```python
from build123d import *

# Parameters (mm, degrees)
SKETCH1_W           = 190
SKETCH1_H           = 114
BOSS_EXTRUDE1_DEPTH = 2.5
SKETCH3_R           = 2
CUT_EXTRUDE2_DEPTH  = 10
SKETCH4_W           = 23
SKETCH4_H           = 13
CUT_EXTRUDE3_DEPTH  = 21


with BuildPart() as part:
    # Sketch1 → Boss-Extrude1 (new body)
    with BuildSketch(Plane.XY):
        Rectangle(SKETCH1_W, SKETCH1_H)
    extrude(amount=BOSS_EXTRUDE1_DEPTH)

    # Sketch3 → Cut-Extrude2 (cut)
    with BuildSketch(Plane.XY.offset(2.5)):
        with Locations((-90, 52)):
            Circle(SKETCH3_R)
        with Locations((90, 52)):
            Circle(SKETCH3_R)
        with Locations((90, -52)):
            Circle(SKETCH3_R)
        with Locations((-90, -52)):
            Circle(SKETCH3_R)
    extrude(amount=-CUT_EXTRUDE2_DEPTH, mode=Mode.SUBTRACT)

    # Sketch4 → Cut-Extrude3 (cut)
    with BuildSketch(Plane.XY.offset(2.5)):
        with Locations((57.5, -39)):
            Rectangle(SKETCH4_W, SKETCH4_H)
    extrude(amount=-CUT_EXTRUDE3_DEPTH, mode=Mode.SUBTRACT)


solid = part.part
```
Work out the finished part from the listing and answer in its coordinate system (mm). Coordinates: 2 decimals unless noted, no trailing zeros. Write each loop counter-clockwise with the first axis right and the second up, starting at its lowest first coordinate (ties: lowest second). Pieces come first, ordered by that corner, then holes.
Q1. A cutting plane is placed at C-C, the plane z = 1.9. Give the vertices of the cut face in (x, y).
Q2. Find the intervals of material crossed by line 1 (Y direction, x = 90, z = 0.9); line 2 (Y direction, x = 56, z = 1.85), in increasing order.
Q3. A cutting plane is placed at D-D, the plane x = -90. Give the vertices of the cut face in (y, z).
Q4. Each of these flat-tipped pins is pushed along its axis until it touches: pin 1 Ø5 at (x, y) = (-90, -52) entering from -Z; pin 2 Ø3 at (x, y) = (90, 52) entering from -Z. Where does it stop, or does it pass through?
Q5. A cutting plane is placed at B-B, the plane y = -52. Give the vertices of the cut face in (x, z).
Q6. Determine the mould class of faces 1 (the face through (-1, 1, 0)), 2 (the face through (91.847, -52.766, 1.268)), 3 (the face through (91.847, 51.234, 1.268)) for opening direction X: released by +X, released by -X, zero draft, split by the parting line, or undercut.
Q7. A cutting plane is placed at A-A, the plane x = 60. Give the vertices of the cut face in (y, z), then the cut area to 4 significant figures.
Findings below:
1. outline: (-95, -57) - (95, -57) - (95, 57) - (-95, 57) - close; hole circle Ø4 at (-90, -52); hole circle Ø4 at (-90, 52); hole (46, -45.5) - (69, -45.5) - (69, -32.5) - (46, -32.5) - close; hole circle Ø4 at (90, -52); hole circle Ø4 at (90, 52)
2. line 1: y = -57 to -54, -50 to 50, 54 to 57
2. line 2: y = -57 to -45.5, -32.5 to 57
3. outline: (-57, 0) - (-54, 0) - (-54, 2.5) - (-57, 2.5) - close; (-50, 0) - (50, 0) - (50, 2.5) - (-50, 2.5) - close; (54, 0) - (57, 0) - (57, 2.5) - (54, 2.5) - close
4. pin 1: stops at z = 0
4. pin 2: passes through
5. outline: (-95, 0) - (-92, 0) - (-92, 2.5) - (-95, 2.5) - close; (-88, 0) - (88, 0) - (88, 2.5) - (-88, 2.5) - close; (92, 0) - (95, 0) - (95, 2.5) - (92, 2.5) - close
6. face 1: zero draft
6. face 2: undercut
6. face 3: undercut
7. outline: (-57, 0) - (-45.5, 0) - (-45.5, 2.5) - (-57, 2.5) - close; (-32.5, 0) - (57, 0) - (57, 2.5) - (-32.5, 2.5) - close
7. area: 252.5 mm2
